Can you work these out from the model? Positions are in its coordinate system, mm. A direction names the side the tool comes from. Give positions to 0.01 mm unless a question says otherwise; leave off trailing zeros. Order: outer loops, then holes, each group sorted by start corner. A loop starts at its lowest first (then second) coordinate and runs counter-clockwise, first axis right, second up. Notation, with made-up numbers: M 21.25,-3 L 42.25,-3 A15 cw 42.25,12 Z; hole C 42.25,5.5 d6. An arc over 180 degrees is marked long. Answer as a JSON object with one key per item and string values.
```python
from build123d import *

# Parameters (mm, degrees)
SKETCH1_W           = 12
SKETCH1_H           = 12
BOSS_EXTRUDE1_DEPTH = 10
FILLET1_R           = 5
SKETCH2_R           = 2
CUT_EXTRUDE1_DEPTH  = 11
SKETCH3_R           = 3.425
CUT_EXTRUDE2_DEPTH  = 6.35


with BuildPart() as part:
    # Sketch1 → Boss-Extrude1 (new body)
    with BuildSketch(Plane(origin=(0, 0, 0), x_dir=(1, 0, 0), z_dir=(0, 1, 0))):
        Rectangle(SKETCH1_W, SKETCH1_H)
    extrude(amount=BOSS_EXTRUDE1_DEPTH)

    # Fillet1
    fillet1_edges = [part.edges().sort_by_distance(p)[0] for p in [
        (-6, 5, -6),
        (6, 5, -6),
        (6, 5, 6),
        (-6, 5, 6),
    ]]
    fillet(fillet1_edges, radius=FILLET1_R)

    # Sketch2 → Cut-Extrude1 (cut, through all)
    with BuildSketch(Plane(origin=(0, 10, 0), x_dir=(1, 0, 0), z_dir=(0, 1, 0))):
        Circle(SKETCH2_R)
    extrude(amount=-CUT_EXTRUDE1_DEPTH, mode=Mode.SUBTRACT)

    # Sketch3 → Cut-Extrude2 (cut)
    with BuildSketch(Plane(origin=(0, 10, 0), x_dir=(1, 0, 0), z_dir=(0, 1, 0))):
        Circle(SKETCH3_R)
    extrude(amount=-CUT_EXTRUDE2_DEPTH, mode=Mode.SUBTRACT)


solid = part.part
```
1) I'm going to push flat-ended pins straight in: pin 1 Ø2 at (x, z) = (-1.5, 0.5) entering from +Y; pin 2 Ø1 at (y, z) = (1.5, 5) entering from -X; pin 3 Ø1.5 at (x, y) = (4, 8.5) entering from -Z. Where does each tip first touch, or does it pass through?
Results found:
{"pin 1": "stops at y = 3.65", "pin 2": "stops at x = -4.57", "pin 3": "stops at z = -5.47"}
2) I want a section at B-B on z = 0. Write out the boundary of the cut face in (x, y) (3 decimals).
Results found:
{"outline": "M -6,0 L -2,0 L -2,3.65 L -3.425,3.65 L -3.425,10 L -6,10 Z; M 2,0 L 6,0 L 6,10 L 3.425,10 L 3.425,3.65 L 2,3.65 Z"}
3) For faces 1 (the face through (0, 3.65, 2.2)), 2 (the face through (0, 5, 6)), which set-ups out of +Z, -Z, +X, -X, +Y, -Y let a thin tool reach every point of the face, with its end or its side?
Results found:
{"face 1": "+Y", "face 2": "+Z, +X, -X, +Y, -Y"}
4) I want a section at A-A on x = 0. Write out the boundary of the cut face in (y, z) (3 decimals).
Results found:
{"outline": "M 0,-6 L 10,-6 L 10,-3.425 L 3.65,-3.425 L 3.65,-2 L 0,-2 Z; M 0,2 L 3.65,2 L 3.65,3.425 L 10,3.425 L 10,6 L 0,6 Z"}
5) I need wall thicknesses on L1, parallel to X at y = 1.25, z = 0; L2, parallel to Z at x = 0, y = 4.25 (3 decimals); L3, parallel to Y at x = -3.25, z = -0.5. Which ranges of each line are inside material? Lowest first, please.
Results found:
{"L1": "x = -6 to -2, 2 to 6", "L2": "z = -6 to -3.425, 3.425 to 6", "L3": "y = 0 to 3.65"}
6) I want a section at D-D on x = 5. Write out the boundary of the cut face in (y, z).
Results found:
{"outline": "M 0,-4 L 10,-4 L 10,4 L 0,4 Z"}
7) I want a section at C-C on y = 0.5. Write out the boundary of the cut face in (x, z), and give its area (3 significant figures).
Results found:
{"outline": "M -6,-1 A5 ccw -1,-6 L 1,-6 A5 ccw 6,-1 L 6,1 A5 ccw 1,6 L -1,6 A5 ccw -6,1 Z; hole C 0,0 d4", "area": "110 mm²"}
8) Thinking about a two-plate mould opening in X: for faces 3 (the face through (-5, 5, 4)), 4 (the face through (0, 5, -6)), 5 (the face through (0, 2, 2)), which applies, pulls with the +X half, pulls with the -X half, needs draft (parallel to the pull), parting line crosses it, or undercut?
Results found:
{"face 3": "pulls with the -X half", "face 4": "needs draft", "face 5": "undercut"}
